Source: CAD feature listing. Evaluate the final solid. Frame: model axes, mm. A direction names the side the tool comes from. Give positions to 0.01 mm unless a question says otherwise; leave off trailing zeros. Write each loop counter-clockwise with the first axis right and the second up, starting at its lowest first coordinate (ties: lowest second). Pieces come first, ordered by that corner, then holes. Notation, with made-up numbers: (48.25, 26.25) - (59.25, 26.25) arc R11 cw to (59.25, 34.25) - close; hole circle Ø9 at (14, -32). An arc over 180 degrees is marked (long way). One line per question, with ' | ' between items. Start each with the question number.
(1) Section B-B, the plane y = 5. Return loops of the section in (x, z).
(2) Access query for faces 1 (the flat face through (23, -21, 2)), 2 (the cylindrical face through (-26.86, 0.55, 7.92)), 3 (the flat face through (12, 20, 12)). Directions: +Z, -Z, +X, -X, +Y, -Y. A direction counts if a zero-diameter tool reaches every point of the face in a straight line with its end or side. Return the directions, or none.
(3) Pin query (flat end, axial travel): pin 1 (12 mm diameter, centred on y = 2, z = 19.5, fed in from -X); pin 2 (3 mm diameter, centred on x = 0, z = 12, fed in from +Y); pin 3 (0.5 mm diameter, centred on x = 12.5, y = -21.5, fed in from -Z). Return the tip coordinate at first contact, or that it passes through.
(4) Section A-A, the plane x = 29. Return loops of the section in (y, z), plus the area to 3 significant figures.
(5) Draft query along X for faces 4 (the flat face through (24, -19, 12)), 5 (the cylindrical face through (-30.5, -12.93, 1.01)), 6 (the flat face through (23, -23.5, 12)). Return one class per face: +X half, -X half, draft (parallel to the pull), parting line (faces both ways), or undercut.
(6) Section C-C, the plane z = 9. State how many separate pieces and enclosed holes the cut face has, plus the area to 3 significant figures.
(7) Section D-D, the plane y = -8. Return loops of the section in (x, z), plus the area to 3 significant figures.
(8) Ray query, line 1 (Y direction, x = -29, z = 0.75); line 2 (Y direction, x = -15, z = 20); line 3 (Y direction, x = -10.5, z = 2.75). Return the intervals inside material, ascending. Write a range as [from, to].
```python
from build123d import *

# Parameters (mm, degrees)
SKETCH_1_W          = 65
SKETCH_1_H          = 37
EXTRUDE_1_DEPTH     = 2
EXTRUDE_2_DEPTH     = 20
SKETCH_3_R          = 6.5
EXTRUDE_3_DEPTH     = 20
SKETCH_4_R          = 12.5
SKETCH_4_R_2        = 6
EXTRUDE_4_DEPTH     = 12
SKETCH_5_W          = 5
SKETCH_5_H          = 10
EXTRUDE_5_DEPTH     = 10
SKETCH_6_R          = 1
EXTRUDE_6_DEPTH     = 1.2
SKETCH_7_W          = 6.798722996
SKETCH_7_H          = 20.12306807
EXTRUDE_7_DEPTH     = 12
CHAMFER_1_SIZE      = 4
SKETCH_8_R          = 1.5
CUT_EXTRUDE_1_DEPTH = 3
SKETCH1_W           = 0.2
SKETCH1_H           = 2.227006651
CUT_EXTRUDE1_DEPTH  = 0.4


with BuildPart() as part:
    # Эскиз1 → Бобышка-Вытянуть1 (new body)
    with BuildSketch(Plane.XY):
        Rectangle(SKETCH_1_W, SKETCH_1_H)
    extrude(amount=EXTRUDE_1_DEPTH)

    # Эскиз2 → Бобышка-Вытянуть2 (add)
    with BuildSketch(Plane.XY.offset(2)):
        Polygon((-24, 23.5), (-24, 13.5), (24, 13.5), (24, 23.5), (22, 23.5), (22, 16), (18, 16), (18, 23.5), (17, 23.5), (17, 16), (13, 16), (13, 23.5), (12, 23.5), (12, 16), (8, 16), (8, 23.5), (7, 23.5), (7, 16), (3, 16), (3, 23.5), (2, 23.5), (2, 16), (-2, 16), (-2, 23.5), (-3, 23.5), (-3, 16), (-7, 16), (-7, 23.5), (-8, 23.5), (-8, 16), (-12, 16), (-12, 23.5), (-13, 23.5), (-13, 16), (-17, 16), (-17, 23.5), (-18, 23.5), (-18, 16), (-22, 16), (-22, 23.5), align=None)
        Polygon((22, -23.5), (24, -23.5), (24, -13.5), (-24, -13.5), (-24, -23.5), (-22, -23.5), (-22, -16), (-18, -16), (-18, -23.5), (-17, -23.5), (-17, -16), (-13, -16), (-13, -23.5), (-12, -23.5), (-12, -16), (-8, -16), (-8, -23.5), (-7, -23.5), (-7, -16), (-3, -16), (-3, -23.5), (-2, -23.5), (-2, -16), (2, -16), (2, -23.5), (3, -23.5), (3, -16), (7, -16), (7, -23.5), (8, -23.5), (8, -16), (12, -16), (12, -23.5), (13, -23.5), (13, -16), (17, -16), (17, -23.5), (18, -23.5), (18, -16), (22, -16), align=None)
    extrude(amount=EXTRUDE_2_DEPTH)

    # Эскиз3 → Бобышка-Вытянуть3 (add)
    with BuildSketch(Plane.XY.offset(2)):
        with Locations((12.5, 6.691570058)):
            Circle(SKETCH_3_R)
        with Locations((12.5, -6.612413993)):
            Circle(SKETCH_3_R)
    extrude(amount=EXTRUDE_3_DEPTH)

    # Эскиз4 → Бобышка-Вытянуть4 (add)
    with BuildSketch(Plane.XY.offset(2)):
        with Locations((-14.373526478, 0)):
            Circle(SKETCH_4_R)
        with Locations((-14.373526478, 0)):
            Circle(SKETCH_4_R_2, mode=Mode.SUBTRACT)
    extrude(amount=EXTRUDE_4_DEPTH)

    # Эскиз5 → Бобышка-Вытянуть5 (add)
    with BuildSketch(Plane.XY.offset(2)):
        with Locations((-29.649429854, 4.142703247)):
            Rectangle(SKETCH_5_W, SKETCH_5_H)
    extrude(amount=EXTRUDE_5_DEPTH)

    # Эскиз6 → Бобышка-Вытянуть6 (add)
    with BuildSketch(Plane.XY.offset(12)):
        with Locations((-30.813495229, 0.582032688)):
            Circle(SKETCH_6_R)
    extrude(amount=EXTRUDE_6_DEPTH)

    # Эскиз7 → Бобышка-Вытянуть7 (add)
    with BuildSketch(Plane.XY.offset(2)):
        with Locations((28.195350692, 0)):
            Rectangle(SKETCH_7_W, SKETCH_7_H)
    extrude(amount=EXTRUDE_7_DEPTH)

    # Фаска1
    chamfer_1_edges = [part.edges().sort_by_distance(p)[0] for p in [
        (31.59471219, 0, 14),
    ]]
    chamfer(chamfer_1_edges, length=CHAMFER_1_SIZE)

    # Эскиз8 → Вырез-Вытянуть1 (cut, through all)
    with BuildSketch(Plane.XY.offset(2)):
        with Locations((-29, 13)):
            Circle(SKETCH_8_R)
        with Locations((29, 13)):
            Circle(SKETCH_8_R)
        with Locations((29, -13)):
            Circle(SKETCH_8_R)
        with Locations((-29, -13)):
            Circle(SKETCH_8_R)
    extrude(amount=-CUT_EXTRUDE_1_DEPTH, mode=Mode.SUBTRACT)

    # Sketch1 → Cut-Extrude1 (cut)
    with BuildSketch(Plane.XY.offset(13.2)):
        with Locations((-30.813495229, 0.505684331)):
            Rectangle(SKETCH1_W, SKETCH1_H)
    extrude(amount=-CUT_EXTRUDE1_DEPTH, mode=Mode.SUBTRACT)


solid = part.part
```
Check sheet entries:
1) outline: (-32.5, 0) - (32.5, 0) - (32.5, 2) - (31.59, 2) - (31.59, 10) - (27.59, 14) - (24.8, 14) - (24.8, 2) - (18.78, 2) - (18.78, 22) - (6.22, 22) - (6.22, 2) - (-2.92, 2) - (-2.92, 14) - (-11.06, 14) - (-11.06, 2) - (-17.69, 2) - (-17.69, 14) - (-25.83, 14) - (-25.83, 2) - (-27.15, 2) - (-27.15, 12) - (-32.15, 12) - (-32.15, 2) - (-32.5, 2) - close
2) face 1: -Z, +X, -X, -Y | face 2: +Z | face 3: +Z, +Y
3) pin 1: x = -26.87 | pin 2: y = 16 | pin 3: z = 2
4) outline: (-18.5, 0) - (-14.5, 0) - (-14.5, 2) - (-18.5, 2) - close; (-11.5, 0) - (11.5, 0) - (11.5, 2) - (10.06, 2) - (10.06, 12.59) - (-10.06, 12.59) - (-10.06, 2) - (-11.5, 2) - close; (14.5, 0) - (18.5, 0) - (18.5, 2) - (14.5, 2) - close | area: 275 mm²
5) face 4: +X half | face 5: undercut | face 6: draft
6) separate pieces: 7 | enclosed holes: 1 | area: 1,250 mm²
7) outline: (-32.5, 0) - (32.5, 0) - (32.5, 2) - (31.59, 2) - (31.59, 10) - (27.59, 14) - (24.8, 14) - (24.8, 2) - (18.85, 2) - (18.85, 22) - (6.15, 22) - (6.15, 2) - (-4.77, 2) - (-4.77, 14) - (-23.98, 14) - (-23.98, 2) - (-32.5, 2) - close | area: 688 mm²
8) line 1: [-18.5, -14.5], [-11.5, 11.5], [14.5, 18.5] | line 2: [-16, -13.5], [13.5, 16] | line 3: [-16, -13.5], [-11.88, -4.58], [4.58, 11.88], [13.5, 16]
